Source: CAD feature listing. Evaluate the final solid. Frame: model axes, mm. A direction names the side the tool comes from. Round coordinates to 2 decimals unless told otherwise and drop trailing zeros. Loops run counter-clockwise (first coordinate to the right, second up) from the corner with the lowest first, then second, coordinate; pieces in that order, holes last.
Item 1: Section query A-A on y = 0. Return loops of the section in (x, z).
Item 2: First-contact query: P1, Ø4, axis at x = -6.5, z = -4, coming from the -Y side; P2, Ø2.5, axis at x = -4.75, y = 8.23, coming from the -Z side; P3, Ø2, axis at y = 1.5, z = 2.5, coming from the -X side; P4, Ø2, axis at x = -3, y = 8, coming from the +Z side. Flat tips, straight axial feed; report the tip coordinate or a pass-through.
Item 3: Section query B-B on x = 0. Return loops of the section in (y, z), then the cut area to 3 significant figures.
Item 4: Pull-direction query (Y, two-part tool) for faces 1 (the flat face through (-3, -1, 4.2)), 2 (the cylindrical face through (-2.75, -12.4, -2.46)), 3 (the cylindrical face through (-5.861, 7.376, -2.465)); classes: released by +Y, released by -Y, zero draft, split by the parting line, or undercut.
Item 5: Ray query, L1, parallel to X at y = 8, z = -0.75; L2, parallel to X at y = -8.5, z = -1; L3, parallel to X at y = -1, z = -3. Return the intervals inside material, ascending.
Item 6: Section query C-C on z = -0.75. Return loops of the section in (x, y), then the cut area to 3 significant figures.
Item 7: Section query D-D on x = 4.75. Return loops of the section in (y, z), then the cut area to 3 significant figures.
Item 8: Access query for faces 4 (the cylindrical face through (4.447, -9.594, -2.465)), 5 (the cylindrical face through (-6, 0, 2)). Directions: +Z, -Z, +X, -X, +Y, -Y. A direction counts if a zero-diameter tool reaches every point of the face in a straight line with its end or side. Return the directions, or none.
```python
from build123d import *

# Parameters (mm, degrees)
SKETCH_1_R           = 12.7
SKETCH_1_R_2         = 1.39954
SKETCH_1_R_3         = 6
EXTRUDE_1_DEPTH      = 5
EXTRUDE_2_DEPTH      = 4.2
EXTRUDE_2_DEPTH_BACK = 5
SKETCH_1_3_R         = 6
SKETCH_1_3_R_2       = 3


with BuildPart() as part:
    # Sketch 1 → Extrude 1 (new body)
    with BuildSketch(Plane.XY):
        Circle(SKETCH_1_R)
        with Locations((4.75, 8.227241336)):
            Circle(SKETCH_1_R_2, mode=Mode.SUBTRACT)
        with Locations((-4.75, 8.227241336)):
            Circle(SKETCH_1_R_2, mode=Mode.SUBTRACT)
        with Locations((-9.5, 0)):
            Circle(SKETCH_1_R_2, mode=Mode.SUBTRACT)
        with Locations((-4.75, -8.227241336)):
            Circle(SKETCH_1_R_2, mode=Mode.SUBTRACT)
        with Locations((4.75, -8.227241336)):
            Circle(SKETCH_1_R_2, mode=Mode.SUBTRACT)
        with Locations((9.5, 0)):
            Circle(SKETCH_1_R_2, mode=Mode.SUBTRACT)
        Circle(SKETCH_1_R_3, mode=Mode.SUBTRACT)
    extrude(amount=-EXTRUDE_1_DEPTH)

    # Sketch 1_3 → Extrude 2 (add, two sides: drawn at the far end of the back side and taken through both)
    with BuildSketch(Plane.XY.offset(-EXTRUDE_2_DEPTH_BACK)):
        Circle(SKETCH_1_3_R)
        Circle(SKETCH_1_3_R_2, mode=Mode.SUBTRACT)
    extrude(amount=EXTRUDE_2_DEPTH + EXTRUDE_2_DEPTH_BACK)


solid = part.part
```
Data:
1. outline: (-12.7, -5) - (-10.9, -5) - (-10.9, 0) - (-12.7, 0) - close; (-8.1, -5) - (-3, -5) - (-3, 4.2) - (-6, 4.2) - (-6, 0) - (-8.1, 0) - close; (3, -5) - (8.1, -5) - (8.1, 0) - (6, 0) - (6, 4.2) - (3, 4.2) - close; (10.9, -5) - (12.7, -5) - (12.7, 0) - (10.9, 0) - close
2. P1: stops at y = -11.88
2. P2: passes through
2. P3: stops at x = -5.98
2. P4: stops at z = 0
3. outline: (-12.7, -5) - (-3, -5) - (-3, 4.2) - (-6, 4.2) - (-6, 0) - (-12.7, 0) - close; (3, -5) - (12.7, -5) - (12.7, 0) - (6, 0) - (6, 4.2) - (3, 4.2) - close
3. area: 122 mm2
4. face 1: zero draft
4. face 2: split by the parting line
4. face 3: undercut
5. L1: x = -9.86 to -6.13, -3.37 to 3.37, 6.13 to 9.86
5. L2: x = -9.44 to -6.12, -3.38 to 3.38, 6.12 to 9.44
5. L3: x = -12.66 to -10.48, -8.52 to -2.83, 2.83 to 8.52, 10.48 to 12.66
6. outline: circle Ø25.4 at (0, 0); hole circle Ø2.8 at (-9.5, 0); hole circle Ø2.8 at (-4.75, -8.23); hole circle Ø2.8 at (-4.75, 8.23); hole circle Ø6 at (0, 0); hole circle Ø2.8 at (4.75, -8.23); hole circle Ø2.8 at (4.75, 8.23); hole circle Ø2.8 at (9.5, 0)
6. area: 442 mm2
7. outline: (-11.78, -5) - (-9.63, -5) - (-9.63, 0) - (-11.78, 0) - close; (-6.83, -5) - (6.83, -5) - (6.83, 0) - (3.67, 0) - (3.67, 4.2) - (-3.67, 4.2) - (-3.67, 0) - (-6.83, 0) - close; (9.63, -5) - (11.78, -5) - (11.78, 0) - (9.63, 0) - close
7. area: 121 mm2
8. face 4: +Z, -Z
8. face 5: +Z
